from build123d import *

# Parameters (mm, degrees)
EXTRUDE_1_DEPTH             = 353
CUT_EXTRUDE_1_REACH         = 91
HOLE_WIZARD_M3_1_AT_2_COUNT = 2
HOLE_WIZARD_M3_1_AT_2_PITCH = 339.768303407
HOLE_WIZARD_M3_1_AT_3_COUNT = 2
HOLE_WIZARD_M3_1_AT_3_PITCH = 340.779254063
HOLE_WIZARD_M3_1_AT_4_COUNT = 2
HOLE_WIZARD_M3_1_AT_4_PITCH = 343.235342003
HOLE_WIZARD_3_2_AT_2_COUNT  = 2
HOLE_WIZARD_3_2_AT_2_PITCH  = 339.809505459
HOLE_WIZARD_3_2_AT_3_COUNT  = 2
HOLE_WIZARD_3_2_AT_3_PITCH  = 343.235342003
HOLE_WIZARD_3_2_AT_4_COUNT  = 2
HOLE_WIZARD_3_2_AT_4_PITCH  = 341.350992382
CUT_EXTRUDE_3_REACH         = 180


with BuildPart() as part:
    # Эскиз1 → Бобышка-Вытянуть1 (new body)
    with BuildSketch(Plane.XY):
        with BuildLine():
            Line((-44.5, -75.5), (-44.5, 75.5))
            ThreePointArc((-44.5, 75.5), (-40.545941546, 85.045941546), (-31, 89))
            Line((-31, 89), (31, 89))
            ThreePointArc((31, 89), (40.545941546, 85.045941546), (44.5, 75.5))
            Line((44.5, 75.5), (44.5, -75.5))
            ThreePointArc((44.5, -75.5), (40.545941546, -85.045941546), (31, -89))
            Line((31, -89), (-31, -89))
            ThreePointArc((-31, -89), (-40.545941546, -85.045941546), (-44.5, -75.5))
        make_face()
        with BuildLine():
            Line((-31, -87.5), (31, -87.5))
            ThreePointArc((31, -87.5), (39.485281374, -83.985281374), (43, -75.5))
            Line((43, -75.5), (43, 75.5))
            ThreePointArc((43, 75.5), (39.485281374, 83.985281374), (31, 87.5))
            Line((31, 87.5), (-31, 87.5))
            ThreePointArc((-31, 87.5), (-39.485281374, 83.985281374), (-43, 75.5))
            Line((-43, 75.5), (-43, -75.5))
            ThreePointArc((-43, -75.5), (-39.485281374, -83.985281374), (-31, -87.5))
        make_face(mode=Mode.SUBTRACT)
    extrude(amount=EXTRUDE_1_DEPTH)

    # Эскиз2 → Вырез-Вытянуть1 (cut, up to next)
    with BuildSketch(Plane(origin=(44.5, 0, 0), x_dir=(0, 0, -1), z_dir=(1, 0, 0)), mode=Mode.PRIVATE) as cut_extrude_1_sk1:
        with BuildLine():
            Line((-266, 3.5), (-92.5, 3.5))
            ThreePointArc((-92.5, 3.5), (-90.378679656, 2.621320344), (-89.5, 0.5))
            Line((-89.5, 0.5), (-89.5, -29.5))
            ThreePointArc((-89.5, -29.5), (-90.378679656, -31.621320344), (-92.5, -32.5))
            Line((-92.5, -32.5), (-266, -32.5))
            ThreePointArc((-266, -32.5), (-268.121320344, -31.621320344), (-269, -29.5))
            Line((-269, -29.5), (-269, 0.5))
            ThreePointArc((-269, 0.5), (-268.121320344, 2.621320344), (-266, 3.5))
        make_face()
    cut_extrude_1_tool1 = extrude(cut_extrude_1_sk1.sketch, amount=-CUT_EXTRUDE_1_REACH, mode=Mode.PRIVATE) & part.part
    add(cut_extrude_1_tool1.solids().sort_by_distance((44.5, -14.5, 179.25))[0], mode=Mode.SUBTRACT)

    # Эскиз4 → M3_впотай_1 (revolve, cut)
    with BuildSketch(Plane(origin=(44.5, 17.5, 345.5), x_dir=(0, 0, -1), z_dir=(0, 1, 0))):
        Polygon((0, 0), (0, 1.5), (2.05, 1.5), (2, 1.45), (2, 1), (3, 0), align=None)
    hole_wizard_m3_1 = revolve(axis=Axis((50.85, 17.5, 345.5), (-1, 0, 0)), mode=Mode.SUBTRACT)

    # M3_впотай_1 at 2: M3_впотай_1 ×2
    with Locations(*[Vector(0, -0.039732959, -0.999210334) * (i * HOLE_WIZARD_M3_1_AT_2_PITCH) for i in range(1, HOLE_WIZARD_M3_1_AT_2_COUNT)]):
        add(hole_wizard_m3_1, mode=Mode.SUBTRACT)

    # M3_впотай_1 at 3: M3_впотай_1 ×2
    with Locations(*[Vector(0, -0.086566303, -0.996246092) * (i * HOLE_WIZARD_M3_1_AT_3_PITCH) for i in range(1, HOLE_WIZARD_M3_1_AT_3_COUNT)]):
        add(hole_wizard_m3_1, mode=Mode.SUBTRACT)

    # M3_впотай_1 at 4: M3_впотай_1 ×2
    with Locations(*[Vector(0, -0.147129371, -0.989117257) * (i * HOLE_WIZARD_M3_1_AT_4_PITCH) for i in range(1, HOLE_WIZARD_M3_1_AT_4_COUNT)]):
        add(hole_wizard_m3_1, mode=Mode.SUBTRACT)

    # Эскиз6 → М3_впотай_2 (revolve, cut)
    with BuildSketch(Plane(origin=(-44.5, 17.5, 345.5), x_dir=(0, 0, 1), z_dir=(0, 1, 0))):
        Polygon((0, 0), (0, 1.5), (2.05, 1.5), (2, 1.45), (2, 1), (3, 0), align=None)
    hole_wizard_3_2 = revolve(axis=Axis((-50.85, 17.5, 345.5), (1, 0, 0)), mode=Mode.SUBTRACT)

    # М3_впотай_2 at 2: М3_впотай_2 ×2
    with Locations(*[Vector(0, -0.042670966, -0.99908918) * (i * HOLE_WIZARD_3_2_AT_2_PITCH) for i in range(1, HOLE_WIZARD_3_2_AT_2_COUNT)]):
        add(hole_wizard_3_2, mode=Mode.SUBTRACT)

    # М3_впотай_2 at 3: М3_впотай_2 ×2
    with Locations(*[Vector(0, -0.147129371, -0.989117257) * (i * HOLE_WIZARD_3_2_AT_3_PITCH) for i in range(1, HOLE_WIZARD_3_2_AT_3_COUNT)]):
        add(hole_wizard_3_2, mode=Mode.SUBTRACT)

    # М3_впотай_2 at 4: М3_впотай_2 ×2
    with Locations(*[Vector(0, -0.103998526, -0.994577451) * (i * HOLE_WIZARD_3_2_AT_4_PITCH) for i in range(1, HOLE_WIZARD_3_2_AT_4_COUNT)]):
        add(hole_wizard_3_2, mode=Mode.SUBTRACT)

    # Эскиз8 → Вырез-Вытянуть3 (cut, up to next)
    with BuildSketch(Plane(origin=(0, 89, 0), x_dir=(1, 0, 0), z_dir=(0, 1, 0)), mode=Mode.PRIVATE) as cut_extrude_3_sk1:
        with BuildLine():
            ThreePointArc((-21.999947808, -282.650594278), (-25.650635095, -312.5), (2.025052192, -324.263114929))
            ThreePointArc((2.025052192, -324.263114929), (10, -324.248711306), (13.999947808, -317.349405722))
            ThreePointArc((13.999947808, -317.349405722), (17.650635095, -287.5), (-10.025052192, -275.736885071))
            ThreePointArc((-10.025052192, -275.736885071), (-18, -275.751288694), (-21.999947808, -282.650594278))
        make_face()
    cut_extrude_3_tool1 = extrude(cut_extrude_3_sk1.sketch, amount=-CUT_EXTRUDE_3_REACH, mode=Mode.PRIVATE) & part.part
    add(cut_extrude_3_tool1.solids().sort_by_distance((-4, 89, 300))[0], mode=Mode.SUBTRACT)

    # Эскиз9 → Зенковка для винта с потайной головкой M41 (revolve, cut)
    with BuildSketch(Plane(origin=(44.5, -12.5, 344), x_dir=(0, 0, -1), z_dir=(0, 1, 0))):
        Polygon((0, 0), (0, 1.5), (2.65, 1.5), (2.6, 1.45), (2.6, 1.15), (3.75, 0), align=None)
    revolve(axis=Axis((50.85, -12.5, 344), (-1, 0, 0)), mode=Mode.SUBTRACT)

    # Эскиз13 → Зенковка для винта с потайной головкой M43 (revolve, cut)
    with BuildSketch(Plane(origin=(-44.5, -12.5, 345.5), x_dir=(0, 0, 1), z_dir=(0, 1, 0))):
        Polygon((0, 0), (0, 1.5), (2.65, 1.5), (2.6, 1.45), (2.6, 1.15), (3.75, 0), align=None)
    revolve(axis=Axis((-50.85, -12.5, 345.5), (1, 0, 0)), mode=Mode.SUBTRACT)


solid = part.part
Here's how the part is built. I have some questions about the finished solid (model axes, mm). A direction names the side the tool comes from. Coordinates: 2 decimals unless noted, no trailing zeros. Order: outer loops, then holes, each group sorted by start corner. A loop starts at its lowest first (then second) coordinate and runs counter-clockwise, first axis right, second up.
Item 1: For P1, Ø1.6, axis at x = 43.5, z = 152, coming from the -Y side (3 decimals); P2, Ø2.5, axis at y = -12, z = 6, coming from the +X side; P3, Ø2.5, axis at y = 4, z = 6, coming from the -X side; P4, Ø3.5, axis at y = -33, z = 6, coming from the -X side, each with a flat end and sliding along its axis, tell me the tip position at first contact or that it passes through.
Result sheet:
P1: stops at y = -82.235
P2: stops at x = -43
P3: stops at x = -43.75
P4: passes through
Item 2: If we mould it in two halves opening along Z, with no side actions, what happens to faces 4 (the face through (0, 89, 174)), 5 (the face through (-17.898, 88.26, 275.694))? For each: +Z half, -Z half, draft (parallel to the pull), parting line (faces both ways), or undercut.
Result sheet:
face 4: draft
face 5: undercut
Item 3: I need wall thicknesses on line 1 (X direction, y = -61.5, z = 14.5); line 2 (Y direction, x = 8, z = 122.5); line 3 (Y direction, x = 43.4, z = 6). Which ranges of each line are inside material? Lowest first, please.
Result sheet:
line 1: x = -44.5 to -43, 43 to 44.5
line 2: y = -89 to -87.5, 87.5 to 89
line 3: y = -80.84 to -35, -31 to -14, -10 to 2, 6 to 80.84
Item 4: If we section it at A-A on x = -14: List the corners of the cut face in (y, z) for me.
Result sheet:
outline: (-89, 0) - (-87.5, 0) - (-87.5, 353) - (-89, 353) - close; (87.5, 0) - (89, 0) - (89, 274.68) - (87.5, 274.68) - close; (87.5, 322.91) - (89, 322.91) - (89, 353) - (87.5, 353) - close
Item 5: If we section it at B-B on y = 10.5: List the corners of the cut face in (x, z) for me.
Result sheet:
outline: (-44.5, 0) - (-43, 0) - (-43, 353) - (-44.5, 353) - close; (43, 0) - (44.5, 0) - (44.5, 353) - (43, 353) - close
Item 6: If we section it at C-C on z = 168: List the corners of the cut face in (x, y) for me.
Result sheet:
outline: (-44.5, -75.5) arc R13.5 ccw to (-31, -89) - (31, -89) arc R13.5 ccw to (44.5, -75.5) - (44.5, -32.5) - (43, -32.5) - (43, -75.5) arc R12 cw to (31, -87.5) - (-31, -87.5) arc R12 cw to (-43, -75.5) - (-43, 75.5) arc R12 cw to (-31, 87.5) - (31, 87.5) arc R12 cw to (43, 75.5) - (43, 3.5) - (44.5, 3.5) - (44.5, 75.5) arc R13.5 ccw to (31, 89) - (-31, 89) arc R13.5 ccw to (-44.5, 75.5) - close
Item 7: If we section it at D-D on z = 60: List the corners of the cut face in (x, y) for me, plus the area to 3 significant figures.
Result sheet:
outline: (-44.5, -75.5) arc R13.5 ccw to (-31, -89) - (31, -89) arc R13.5 ccw to (44.5, -75.5) - (44.5, 75.5) arc R13.5 ccw to (31, 89) - (-31, 89) arc R13.5 ccw to (-44.5, 75.5) - close; hole (-43, -75.5) arc R12 ccw to (-31, -87.5) - (31, -87.5) arc R12 ccw to (43, -75.5) - (43, 75.5) arc R12 ccw to (31, 87.5) - (-31, 87.5) arc R12 ccw to (-43, 75.5) - close
area: 759 mm2
Item 8: For faces 1 (the face through (-39.58, -83.89, 174.03)), 2 (the face through (-25.87, 88.26, 312.11)), 3 (the face through (0, -89, 174)), which set-ups out of +Z, -Z, +X, -X, +Y, -Y let a thin tool reach every point of the face, with its end or its side?
Result sheet:
face 1: +Z, -Z
face 2: +Y
face 3: +Z, -Z, +X, -X, -Y
